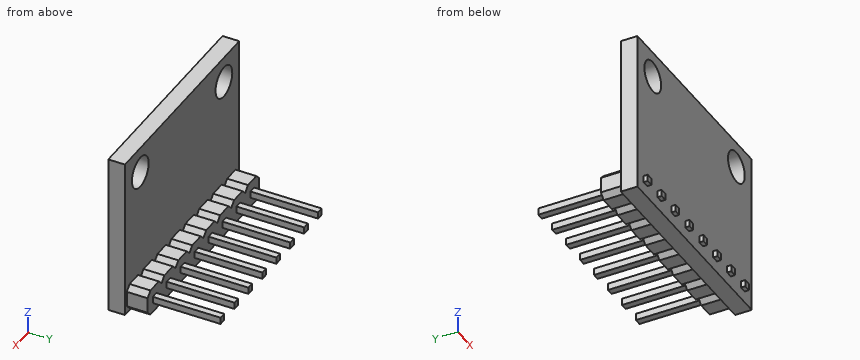
from build123d import *

# Parameters (mm, degrees)
SKETCH1_W           = 20.5
SKETCH1_H           = 15.6
SKETCH1_R           = 1.5
BOSS_EXTRUDE1_DEPTH = 1.6
BOSS_EXTRUDE2_DEPTH = 2
BOSS_EXTRUDE3_START = -4
SKETCH3_W           = 0.65
SKETCH3_H           = 0.65
BOSS_EXTRUDE3_DEPTH = 10.5
LPATTERN1_COUNT     = 8
LPATTERN1_PITCH     = 2.5


with BuildPart() as part:
    # Sketch1 → Boss-Extrude1 (new body)
    with BuildSketch(Plane(origin=(0, 0, 0), x_dir=(1, 0, 0), z_dir=(0, 1, 0))):
        with Locations((0, 7.8)):
            Rectangle(SKETCH1_W, SKETCH1_H)
        with Locations(Location((7.5, 2.5, 0), (0, 0, 270))):
            Circle(SKETCH1_R, mode=Mode.SUBTRACT)
        with Locations(Location((-7.5, 2.5, 0), (0, 0, 90))):
            Circle(SKETCH1_R, mode=Mode.SUBTRACT)
    extrude(amount=BOSS_EXTRUDE1_DEPTH)

    # Sketch2 → Boss-Extrude2 (add)
    with BuildSketch(Plane(origin=(0, 1.6, 0), x_dir=(1, 0, 0), z_dir=(0, 1, 0))):
        Polygon((7.918720213, 15.4), (7.418720213, 14.9), (6.918720213, 15.4), (5.418720213, 15.4), (4.918720213, 14.9), (4.418720213, 15.4), (2.918720213, 15.4), (2.418720213, 14.9), (1.918720213, 15.4), (0.418720213, 15.4), (-0.081279787, 14.9), (-0.581279787, 15.4), (-2.081279787, 15.4), (-2.581279787, 14.9), (-3.081279787, 15.4), (-4.581279787, 15.4), (-5.081279787, 14.9), (-5.581279787, 15.4), (-7.081279787, 15.4), (-7.581279787, 14.9), (-8.081279787, 15.4), (-9.581279787, 15.4), (-10.081279787, 14.9), (-10.081279787, 13.4), (-9.581279787, 12.9), (-8.081279787, 12.9), (-7.581279787, 13.4), (-7.081279787, 12.9), (-5.581279787, 12.9), (-5.081279787, 13.4), (-4.581279787, 12.9), (-3.081279787, 12.9), (-2.581279787, 13.4), (-2.081279787, 12.9), (-0.581279787, 12.9), (-0.081279787, 13.4), (0.418720213, 12.9), (1.918720213, 12.9), (2.418720213, 13.4), (2.918720213, 12.9), (4.418720213, 12.9), (4.918720213, 13.4), (5.418720213, 12.9), (6.918720213, 12.9), (7.418720213, 13.4), (7.918720213, 12.9), (9.418720213, 12.9), (9.918720213, 13.4), (9.918720213, 14.9), (9.418720213, 15.4), align=None)
    extrude(amount=BOSS_EXTRUDE2_DEPTH)

    # Sketch3 → Boss-Extrude3 (add)
    with BuildSketch(Plane(origin=(0, 3.6, 0), x_dir=(1, 0, 0), z_dir=(0, 1, 0)).offset(BOSS_EXTRUDE3_START)):
        with Locations((8.668720213, 14.15)):
            Rectangle(SKETCH3_W, SKETCH3_H)
    boss_extrude3 = extrude(amount=BOSS_EXTRUDE3_DEPTH)

    # LPattern1: Boss-Extrude3 ×8
    with Locations(*[(-i * LPATTERN1_PITCH, 0, 0) for i in range(1, LPATTERN1_COUNT)]):
        add(boss_extrude3)


solid = part.part
CAD build for the part. Positions are in the model's coordinates, mm. Round coordinates to 2 decimals unless told otherwise and drop trailing zeros. Write each loop counter-clockwise with the first axis right and the second up, starting at its lowest first coordinate (ties: lowest second). Pieces come first, ordered by that corner, then holes. Notation, with made-up numbers: M -7.5,-31.5 L 50.5,-31.5 A30 ccw 50.5,-3.5 Z; hole C 25.25,79 d2. An arc over 180 degrees is marked long. Put each result on its own line as item: value. Start each with the question number.
1) Drill centre lines: probe 1 along X at (y, z) = (0.95, -2.5); probe 2 along Z at (x, y) = (-7.5, 1.15); probe 3 along Y at (x, z) = (-5.25, -4.75). Where is each one in solid material? Low to high. Write a range as [from, to].
2) Pin check, flat tips, straight feed: pin 1 Ø2 at (x, z) = (7, -11.5) entering from -Y; pin 2 Ø1 at (x, y) = (-6.5, 3) entering from -Z; pin 3 Ø2 at (y, z) = (3.5, -7) entering from -X; pin 4 Ø0.7 at (y, z) = (6.5, -14) entering from -X. Stop position of each tip, or through.
3) Saw through at C-C, the plane x = -1.25. Write the cut outline in (y, z) (3 decimals).
4) Saw through at A-A, the plane z = -2.5. Write the cut outline in (x, y).
5) Saw through at D-D, the plane z = -7. Write the cut outline in (x, y), and give its area (3 significant figures).
6) Saw through at B-B, the plane y = 8.5. Count the separate pieces of the cut face and the enclosed holes in it, and give its area (3 significant figures).
Resolved:
1. probe 1: [-10.25, -9], [-6, 6], [9, 10.25]
1. probe 2: [-15.6, -4], [-1, 0]
1. probe 3: [0, 1.6]
2. pin 1: y = 0
2. pin 2: z = -15.4
2. pin 3: through
2. pin 4: x = -9.16
3. outline: M -0.4,-14.475 L 0,-14.475 L 0,-15.6 L 1.6,-15.6 L 1.6,-15.4 L 3.6,-15.4 L 3.6,-14.475 L 10.1,-14.475 L 10.1,-13.825 L 3.6,-13.825 L 3.6,-12.9 L 1.6,-12.9 L 1.6,0 L 0,0 L 0,-13.825 L -0.4,-13.825 Z
4. outline: M -10.25,0 L -9,0 L -9,1.6 L -10.25,1.6 Z; M -6,0 L 6,0 L 6,1.6 L -6,1.6 Z; M 9,0 L 10.25,0 L 10.25,1.6 L 9,1.6 Z
5. outline: M -10.25,0 L 10.25,0 L 10.25,1.6 L -10.25,1.6 Z
5. area: 32.8 mm²
6. separate pieces: 8
6. enclosed holes: 0
6. area: 3.38 mm²
